Input: part model. Units: mm. Frame: model coordinates. Face numbers are marked on the shaded views. A direction names the side the tool comes from. Give positions to 0.01 mm unless a question says otherwise; leave off trailing zeros.
```python
from build123d import *

# Parameters (mm, degrees)
F0_W     = 22
F0_H     = 25.2
F1_DEPTH = 9.75
F3_DEPTH = 25.2
F12_R    = 2
F13_R    = 0.75


with BuildPart() as f1:
    # F0 (on Top) → F1 (new body)
    with BuildSketch(Plane.XY):
        Rectangle(F0_W, F0_H)
    extrude(amount=F1_DEPTH)

    # F2 (on face) → F3 (cut, through all)
    with BuildSketch(Plane.XZ.offset(12.6)):
        Polygon((-8, 2.875), (-8, 6.875), (-11, 7.75), (-11, 2), align=None)
        Polygon((11, 7.75), (8, 6.875), (8, 2.875), (11, 2), align=None)
    extrude(amount=-F3_DEPTH, mode=Mode.SUBTRACT)

    # F4 (on Right) → F5 (revolve, cut)
    with BuildSketch(Plane.YZ):
        with BuildLine():
            Line((0, 9.75), (0, 6.75))
            Line((0, 6.75), (4.3, 6.75))
            ThreePointArc((4.3, 6.75), (6.914658, 7.981058), (9.2, 9.75))
            Line((9.2, 9.75), (0, 9.75))
        make_face()
    revolve(axis=Axis((0, 0, 8.25), (0, 0, -1)), mode=Mode.SUBTRACT)

    # F6 (on Front) → F7 (revolve, cut)
    with BuildSketch(Plane.XZ):
        with BuildLine():
            Line((0, -1.25), (6.1, -1.25))
            ThreePointArc((6.1, -1.25), (5.667858, 5.198602), (0, 8.3045))
            Line((0, 8.3045), (0, -1.25))
        make_face()
    revolve(axis=Axis((0, 0, 3.52725), (0, 0, -1)), mode=Mode.SUBTRACT)

    # F6 (on Front) → F10 (revolve, cut)
    with BuildSketch(Plane.XZ):
        with BuildLine():
            Line((0, -1.25), (6.1, -1.25))
            ThreePointArc((6.1, -1.25), (5.667858, 5.198602), (0, 8.3045))
            Line((0, 8.3045), (0, -1.25))
        make_face()
    revolve(axis=Axis((0, 0, 3.490293), (0, 0, -1)), mode=Mode.SUBTRACT)

    # F8 (on Front) → F11 (revolve)
    with BuildSketch(Plane.XZ):
        with BuildLine():
            ThreePointArc((6.536245, 0), (6.34896, -0.635762), (6.1, -1.25))
            ThreePointArc((6.1, -1.25), (8.323498, -0.707714), (10.5, 0))
            Line((10.5, 0), (6.536245, 0))
        make_face()
    revolve(axis=Axis((0, 0, 3.52725), (0, 0, -1)))

    # F12
    f12_edges = [f1.edges().sort_by_distance(p)[0] for p in [
        (-10.5, 0, 0),
    ]]
    fillet(f12_edges, radius=F12_R)

    # F13
    f13_edges = [f1.edges().sort_by_distance(p)[0] for p in [
        (8, 0, 2.875),
        (8, 0, 6.875),
        (-8, 0, 6.875),
        (-8, 0, 2.875),
    ]]
    fillet(f13_edges, radius=F13_R)


solid = f1.part
```
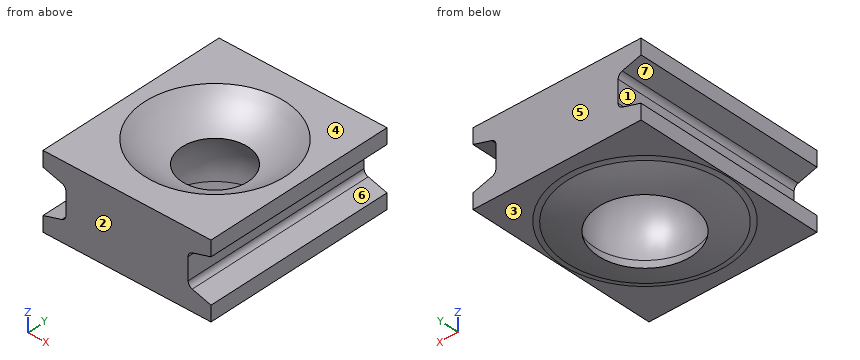
Item 1: Pin query (flat end, axial travel): pin 1 (1 mm diameter, centred on x = 0, y = -8, fed in from -Z); pin 2 (2.5 mm diameter, centred on y = -3, z = 4.5, fed in from +X); pin 3 (2.5 mm diameter, centred on y = -0.5, z = 5, fed in from -X). Return the tip coordinate at first contact, or that it passes through.
Item 2: Ray query, line 1 (X direction, y = -6.5, z = 6); line 2 (Y direction, x = -5.75, z = 2.25); line 3 (Z direction, x = -3, y = -10.75). Return the intervals inside material, ascending.
Item 3: Set-up query: the marked faces 5, 6 and 7. Return all of +Z, -Z, +X, -X, +Y, -Y with unobstructed straight access to the full face (end or side cutting, diameter ignored); none if empty.
Item 4: Mould query, pull axis Z, two halves, no side actions, for the marked faces 1, 2, 3 and 4. Classes: +Z half, -Z half, draft (parallel to the pull), parting line (faces both ways), or undercut.
Solved:
1. pin 1: stops at z = -0.93
1. pin 2: stops at x = 8.02
1. pin 3: stops at x = -8
2. line 1: x = -8 to 8
2. line 2: y = -12.6 to -3.42, 3.42 to 12.6
2. line 3: z = 0 to 9.75
3. face 5: +Z, -Z, +X, -X, +Y
3. face 6: +X, +Y, -Y
3. face 7: -X, +Y, -Y
4. face 1: undercut
4. face 2: draft
4. face 3: -Z half
4. face 4: +Z half
